The model under review builds one solid part; all positions refer to its coordinate system, in mm. A direction names the side the tool comes from. Coordinates: 2 decimals unless noted, no trailing zeros. Write each loop counter-clockwise with the first axis right and the second up, starting at its lowest first coordinate (ties: lowest second). Pieces come first, ordered by that corner, then holes.
Autodesk Inventor part; units mm, degrees
ref_plane "YZ Plane" through (0, 0, 0) normal (1, 0, 0) x (0, 1, 0)
ref_plane "XZ Plane" through (0, 0, 0) normal (0, 1, 0) x (-1, 0, 0)
ref_plane "XY Plane" through (0, 0, 0) normal (0, 0, 1) x (1, 0, 0)
sketch "Sketch1" plane through (0, 0, 0) normal (0, 1, 0) x (-1, 0, 0)
  circle A0 centre (0, 0) radius 11.43
  circle A1 centre (0, 0) radius 9.525
  dimension "d0" = 19.05
  dimension "d1" = 22.86
extrude "Extrusion1" add sketch "Sketch1" along normal blind 12.7
sketch "Sketch2" plane through (0, 12.7, 0) normal (0, 1, 0) x (1, 0, 0)
  point P0 (0, 0)
sketch "Sketch3" plane through (0, 0, 0) normal (1, 0, 0) x (0, 1, 0)
  line L0 (12.7, -11.43) -> (12.7, 11.43)
  line L1 (12.7, 1.5875) -> (6.35, 1.5875)
  line L2 (6.35, -1.5875) -> (12.7, -1.5875)
  line L3 (12.7, 1.5875) -> (12.7, -1.5875)
  arc A0 (6.35, 1.5875) -> (6.35, -1.5875) centre (6.35, 0) ccw
  point P0 (0, 0)
  point P1 (9.525, -1.5875)
  point P2 (12.7, 0)
  dimension "d4" = 3.175
  dimension "d5" = 6.35
extrude "Extrusion2" cut sketch "Sketch3" against normal blind 12.7
properties part number "smallinsert1"
Item 1: Machinability: for faces 1 (the face through (-10.397, 4.763, 0.035)), 2 (the face through (7.559, 6.261, 5.796)), which of the approach directions +Z, -Z, +X, -X, +Y, -Y give a long, thin tool a straight path to every point of the face, cutting with its end or side? Answer none if there is none.
Solved:
face 1: -X, +Y
face 2: +Y, -Y
Item 2: For pin 1 (1 mm diameter, centred on x = -6.5, y = 7, fed in from -Z); pin 2 (5 mm diameter, centred on y = 9.5, z = -3, fed in from -X); pin 3 (1 mm diameter, centred on x = -2.5, y = 2, fed in from +Z); pin 4 (1 mm diameter, centred on x = 6.5, z = 3, fed in from +Y), all flat-tipped, find the tip position at first contact; note any pin that passes through.
Solved:
pin 1: stops at z = -9.73
pin 2: stops at x = -11.32
pin 3: stops at z = 11.25
pin 4: passes through
Item 3: Mouldability with a two-part tool opening along Z and no side actions: class faces 3 (the face through (9, 12.7, 4)), 4 (the face through (-10, 9, -1.588)), 5 (the face through (-10.902, 6.261, -3.433)) as pulls with the +Z half, pulls with the -Z half, needs draft (parallel to the pull), parting line crosses it, or undercut.
Solved:
face 3: needs draft
face 4: undercut
face 5: parting line crosses it
Item 4: To check wall thickness, follow line 1 along Z through (x, y) = (0, 3.75) (3 decimals); line 2 along X through (y, z) = (7.75, 0) (3 decimals). State the ranges of each line that lie inside material, in increasing order.
Solved:
line 1: z = -11.43 to -9.525, 9.525 to 11.43
line 2: x = 9.525 to 11.43
Item 5: Take a section at D-D, the plane y = 2. Write out the cut boundary in (x, z) (3 decimals).
Solved:
outline: circle Ø22.86 at (0, 0); hole circle Ø19.05 at (0, 0)
Item 6: Take a section at A-A, the plane x = 0. Write out the cut boundary in (y, z) (3 decimals), plus the area to 3 significant figures.
Solved:
outline: (0, -11.43) - (12.7, -11.43) - (12.7, -9.525) - (0, -9.525) - close; (0, 9.525) - (12.7, 9.525) - (12.7, 11.43) - (0, 11.43) - close
area: 48.4 mm2
Item 7: Take a section at B-B, the plane z = 0. Write out the cut boundary in (x, y) (1 decimal).
Solved:
outline: (-11.4, 0) - (-9.5, 0) - (-9.5, 4.8) - (-11.4, 4.8) - close; (9.5, 0) - (11.4, 0) - (11.4, 12.7) - (9.5, 12.7) - close
